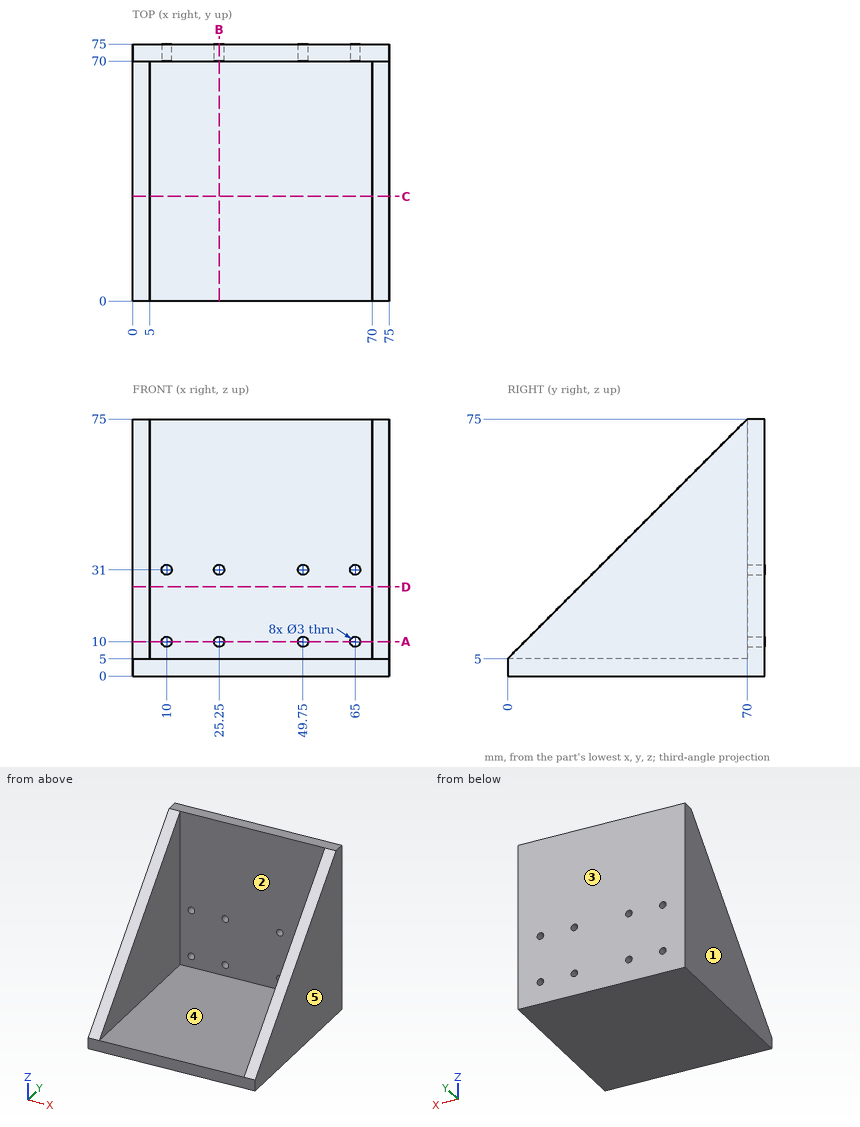
The figure shows three views and two pictorial views of one solid part (mm, origin at its lowest corner). Answer the questions. A direction names the side the tool comes from. Round coordinates to 2 decimals unless told otherwise and drop trailing zeros. Loops run counter-clockwise (first coordinate to the right, second up) from the corner with the lowest first, then second, coordinate; pieces in that order, holes last. Notation, with made-up numbers: M 42,-6.5 L 65,-6.5 A15 ccw 65,7.5 Z; hole C 50,42.25 d5. An arc over 180 degrees is marked long. Return JSON: item names as keys, results as strings.
Q1. Find section B-B, the plane x = 25.25. Determine the outline of the cut face in (y, z), plus the area to 3 significant figures.
Results list:
{"outline": "M 0,0 L 75,0 L 75,8.5 L 70,8.5 L 70,5 L 0,5 Z; M 70,11.5 L 75,11.5 L 75,29.5 L 70,29.5 Z; M 70,32.5 L 75,32.5 L 75,75 L 70,75 Z", "area": "695 mm2"}
Q2. The mould has two halves that part along X. Classify the marked faces 1, 2 and 3: released by +X, released by -X, zero draft, split by the parting line, or undercut.
Results list:
{"face 1": "released by -X", "face 2": "undercut", "face 3": "zero draft"}
Q3. Find section A-A, the plane z = 10. Determine the outline of the cut face in (x, y), plus the area to 3 significant figures.
Results list:
{"outline": "M 0,5 L 5,5 L 5,70 L 8.5,70 L 8.5,75 L 0,75 Z; M 11.5,70 L 23.75,70 L 23.75,75 L 11.5,75 Z; M 26.75,70 L 48.25,70 L 48.25,75 L 26.75,75 Z; M 51.25,70 L 63.5,70 L 63.5,75 L 51.25,75 Z; M 66.5,70 L 70,70 L 70,5 L 75,5 L 75,75 L 66.5,75 Z", "area": "965 mm2"}
Q4. Find section D-D, the plane z = 26. Determine the outline of the cut face in (x, y), plus the area to 3 significant figures.
Results list:
{"outline": "M 0,21 L 5,21 L 5,70 L 70,70 L 70,21 L 75,21 L 75,75 L 0,75 Z", "area": "865 mm2"}
Q5. Each of these flat-tipped pins is pushed along its axis until it touches: pin 1 Ø2.5 at (x, z) = (65, 10) entering from -Y; pin 2 Ø1 at (x, y) = (43, 22) entering from +Z; pin 3 Ø19.5 at (x, z) = (23, 34.5) entering from -Y. Where does it stop, or does it pass through?
Results list:
{"pin 1": "passes through", "pin 2": "stops at z = 5", "pin 3": "stops at y = 70"}
Q6. Find the intervals of material crossed by line 1 along Z through (x, y) = (25.25, 73.5); line 2 along X through (y, z) = (59.5, 27.5); line 3 along Y through (x, z) = (63.5, 67), in increasing order. Write a range as from..to.
Results list:
{"line 1": "z = 0..8.5, 11.5..29.5, 32.5..75", "line 2": "x = 0..5, 70..75", "line 3": "y = 70..75"}
Q7. Which of the six approach directions +Z, -Z, +X, -X, +Y, -Y give full straight-line access (tool end or side, diameter ignored) to the marked faces 4 and 5?
Results list:
{"face 4": "+Z, -Y", "face 5": "+Z, -Z, +X, +Y, -Y"}
Q8. Find section C-C, the plane y = 30.5. Determine the outline of the cut face in (x, z), plus the area to 3 significant figures.
Results list:
{"outline": "M 0,0 L 75,0 L 75,35.5 L 70,35.5 L 70,5 L 5,5 L 5,35.5 L 0,35.5 Z", "area": "680 mm2"}
